Can you work these out from the model? Positions are in its coordinate system, mm. A direction names the side the tool comes from. Round coordinates to 2 decimals unless told otherwise and drop trailing zeros. Order: outer loops, then holes, each group sorted by start corner. A loop starts at its lowest first (then second) coordinate and runs counter-clockwise, first axis right, second up. Notation, with made-up numbers: (70.25, 40) - (85.25, 40) arc R18 cw to (85.25, 61) - close; hole circle Ø1 at (33.25, -12.5). An arc over 180 degrees is marked (long way). Write item = value, one per line.
from build123d import *

# Parameters (mm, degrees)
SKETCH2_R           = 8
BOSS_EXTRUDE1_DEPTH = 1.6
FILLET1_R           = 0.635
FILLET2_R           = 1.27


with BuildPart() as part:
    # Sketch2 → Boss-Extrude1 (new body)
    with BuildSketch(Plane.XY):
        with BuildLine():
            Line((-5.5, 32.016485365), (-5.5, 41.221120861))
            Line((-5.5, 41.221120861), (5.5, 41.221120861))
            Line((5.5, 41.221120861), (5.5, 32.016485365))
            ThreePointArc((5.5, 32.016485365), (11.977775563, 22.081115767), (6.7545, 11.43261645))
            Line((6.7545, 11.43261645), (6.7545, 4.296230906))
            Line((6.7545, 4.296230906), (3, 4.296230906))
            ThreePointArc((3, 4.296230906), (5.219764516, 0.460063475), (3.705239533, -3.705239533))
            Line((3.705239533, -3.705239533), (2.644579362, -2.644579362))
            ThreePointArc((2.644579362, -2.644579362), (3.596344694, 1.026598676), (0.85, 3.642128499))
            Line((0.85, 3.642128499), (0.85, 0.74))
            Line((0.85, 0.74), (-0.85, 0.74))
            Line((-0.85, 0.74), (-0.85, 3.642128499))
            ThreePointArc((-0.85, 3.642128499), (-3.596344694, 1.026598676), (-2.644579362, -2.644579362))
            Line((-2.644579362, -2.644579362), (-3.705239533, -3.705239533))
            ThreePointArc((-3.705239533, -3.705239533), (-5.219764516, 0.460063475), (-3, 4.296230906))
            Line((-3, 4.296230906), (-6.7545, 4.296230906))
            Line((-6.7545, 4.296230906), (-6.7545, 11.43261645))
            ThreePointArc((-6.7545, 11.43261645), (-11.977775563, 22.081115767), (-5.5, 32.016485365))
        make_face()
        with Locations((0, 21.351120861)):
            Circle(SKETCH2_R, mode=Mode.SUBTRACT)
        with BuildLine():
            Line((-2.75, 39.221120861), (2.75, 39.221120861))
            Line((2.75, 39.221120861), (2.75, 33.031767248))
            ThreePointArc((2.75, 33.031767248), (0, 33.351120861), (-2.75, 33.031767248))
            Line((-2.75, 33.031767248), (-2.75, 39.221120861))
        make_face(mode=Mode.SUBTRACT)
        Polygon((-1.25, 6.796230906), (-1.25, 8.796230906), (1.25, 8.796230906), (1.25, 6.796230906), (4.2545, 6.796230906), (4.2545, 11.196230906), (-4.2545, 11.196230906), (-4.2545, 6.796230906), align=None, mode=Mode.SUBTRACT)
    extrude(amount=BOSS_EXTRUDE1_DEPTH)

    # Fillet1
    fillet1_edges = [part.edges().sort_by_distance(p)[0] for p in [
        (-3, 4.296230906, 0.8),
        (3, 4.296230906, 0.8),
    ]]
    fillet(fillet1_edges, radius=FILLET1_R)

    # Fillet2
    fillet2_edges = [part.edges().sort_by_distance(p)[0] for p in [
        (-6.7545, 4.296230906, 0.8),
        (-6.7545, 11.43261645, 0.8),
        (-5.5, 32.016485365, 0.8),
        (-5.5, 41.221120861, 0.8),
        (5.5, 41.221120861, 0.8),
        (5.5, 32.016485365, 0.8),
        (6.7545, 11.43261645, 0.8),
        (6.7545, 4.296230906, 0.8),
        (3.705239533, -3.705239533, 0.8),
        (-3.705239533, -3.705239533, 0.8),
    ]]
    fillet(fillet2_edges, radius=FILLET2_R)


solid = part.part
(1) If we section it at B-B (y = 35): Write out the boundary of the cut face in (x, z), plus the area to 3 significant figures.
Computed:
outline = (-5.5, 0) - (-2.75, 0) - (-2.75, 1.6) - (-5.5, 1.6) - close; (2.75, 0) - (5.5, 0) - (5.5, 1.6) - (2.75, 1.6) - close
area = 8.80 mm^2
(2) If we section it at C-C (y = 28.5): Write out the boundary of the cut face in (x, z), plus the area to 3 significant figures.
Computed:
outline = (-9.64, 0) - (-3.59, 0) - (-3.59, 1.6) - (-9.64, 1.6) - close; (3.59, 0) - (9.64, 0) - (9.64, 1.6) - (3.59, 1.6) - close
area = 19.4 mm^2
(3) On a 3-axis mill with a long thin cutter (end or side, diameter ignored), from which of +Z, -Z, +X, -X, +Y, -Y can I reach the whole of each face in a straight line? I mean faces 1 (the face through (-0.85, 2, 1)), 2 (the face through (-5, 4.296, 1)), 3 (the face through (2.75, 36, 1)), 4 (the face through (6.392, 4.678, 0.811)). Say none if no direction works.
Computed:
face_1 = +Z, -Z, -Y
face_2 = +Z, -Z, -X
face_3 = +Z, -Z
face_4 = +Z, -Z, +X, -Y
(4) If we section it at D-D (z = 1.15): State how many separate pieces and enclosed holes the cut face has, plus the area to 3 significant figures.
Computed:
separate_pieces = 1
enclosed_holes = 3
area = 386 mm^2
(5) If we section it at A-A (x = 0): Write out the boundary of the cut face in (y, z), plus the area to 3 significant figures.
Computed:
outline = (0.74, 0) - (8.8, 0) - (8.8, 1.6) - (0.74, 1.6) - close; (11.2, 0) - (13.35, 0) - (13.35, 1.6) - (11.2, 1.6) - close; (29.35, 0) - (33.35, 0) - (33.35, 1.6) - (29.35, 1.6) - close; (39.22, 0) - (41.22, 0) - (41.22, 1.6) - (39.22, 1.6) - close
area = 25.9 mm^2
(6) Thinking about a two-plate mould opening in Y: for faces 5 (the face through (5, 4.296, 1)), 6 (the face through (11.97, 22.2, 0.79)), 7 (the face through (-5.67, 32.13, 0.81)), which applies, +Y half, -Y half, draft (parallel to the pull), parting line (faces both ways), or undercut?
Computed:
face_5 = undercut
face_6 = parting line
face_7 = +Y half
(7) If I drill on line 1 (Y direction, x = -0.25, z = 0.35); line 2 (X direction, y = 28, z = 0.65); line 3 (X direction, y = 25, z = 1.2), over which ranges is the centre line in solid material (lowest first)? Write a range as from..to.
Computed:
line_1 = 0.74..8.8, 11.2..13.36, 29.35..33.35, 39.22..41.22
line_2 = -9.99..-4.45, 4.45..9.99
line_3 = -11.43..-7.12, 7.12..11.43
(8) Will these pins go through, and if not, where does the flat tip stop? P1, Ø0.7, axis at x = 5, z = 0.5, coming from the -Y side; P2, Ø0.5, axis at y = 37, z = 1, coming from the +X side; P3, Ø0.5, axis at y = 1.5, z = 0.5, coming from the -X side.
Computed:
P1 = -2.41
P2 = 5.5
P3 = -5.09
